from build123d import *

# Parameters (mm, degrees)
SKETCH1_W                    = 100
SKETCH1_H                    = 214.69
BASE_FLANGE1_DEPTH           = 0.81
EDGE_FLANGE1_STRIP_W         = 4.7132
EDGE_FLANGE1_STRIP_H         = 0.81
EDGE_FLANGE1_STRIP_CUT_DEPTH = 214.69
EDGE_FLANGE1_DEPTH           = 214.69
EDGE_FLANGE2_STRIP_W         = 4.7132
EDGE_FLANGE2_STRIP_H         = 0.81
EDGE_FLANGE2_STRIP_CUT_DEPTH = 214.69
EDGE_FLANGE2_DEPTH           = 214.69
EDGE_FLANGE3_DEPTH           = 98.4534
EDGE_FLANGE3_BEND_DEPTH      = 97.2634
SKETCH18_W                   = 29
SKETCH18_H                   = 1.5466
SKETCH18_W_2                 = 27
CUT_EXTRUDE1_DEPTH           = 23.81
CUT_EXTRUDE2_REACH           = 249.484
SKETCH19_R                   = 2.5
SKETCH19_R_2                 = 3.5
SKETCH19_R_3                 = 1.5
SKETCH19_R_4                 = 3.25
CUT_EXTRUDE3_REACH           = 249.484
SKETCH20_R                   = 1.85
SKETCH20_R_2                 = 2.5
SKETCH20_R_3                 = 3.5


# Sheet-metal steps are written as plain solids
with BuildPart() as part:
    # Sketch1 → Base-Flange1 (new body)
    with BuildSketch(Plane.XY):
        with Locations((50, 107.345)):
            Rectangle(SKETCH1_W, SKETCH1_H)
    extrude(amount=-BASE_FLANGE1_DEPTH)

    # Edge-Flange1 strip (across the edge) → Edge-Flange1 strip cut (cut)
    with BuildSketch(Plane(origin=(100, 214.69, -0.81), x_dir=(-1, 0, 0), z_dir=(0, -1, 0))):
        with Locations((-0.81, -0.405)):
            Rectangle(EDGE_FLANGE1_STRIP_W, EDGE_FLANGE1_STRIP_H)
    extrude(amount=EDGE_FLANGE1_STRIP_CUT_DEPTH, mode=Mode.SUBTRACT)

    # Edge-Flange1 section (across the edge) → Edge-Flange1 (add)
    with BuildSketch(Plane(origin=(100, 214.69, -0.81), x_dir=(-1, 0, 0), z_dir=(0, -1, 0))):
        with BuildLine():
            Line((0, 0.7366), (0, 48))
            Line((0, 48), (0.81, 48))
            Line((0.81, 48), (0.81, 0.7366))
            ThreePointArc((0.81, 0.7366), (1.025745145, 0.215745145), (1.5466, 0))
            Line((1.5466, 0), (1.5466, -0.81))
            ThreePointArc((1.5466, -0.81), (0.452988652, -0.357011348), (0, 0.7366))
        make_face()
    extrude(amount=EDGE_FLANGE1_DEPTH)

    # Edge-Flange2 strip (across the edge) → Edge-Flange2 strip cut (cut)
    with BuildSketch(Plane(origin=(99.19, 214.69, -48.81), x_dir=(0, 0, 1), z_dir=(0, -1, 0))):
        with Locations((-0.81, -0.405)):
            Rectangle(EDGE_FLANGE2_STRIP_W, EDGE_FLANGE2_STRIP_H)
    extrude(amount=EDGE_FLANGE2_STRIP_CUT_DEPTH, mode=Mode.SUBTRACT)

    # Edge-Flange2 section (across the edge) → Edge-Flange2 (add)
    with BuildSketch(Plane(origin=(99.19, 214.69, -48.81), x_dir=(0, 0, 1), z_dir=(0, -1, 0))):
        with BuildLine():
            Line((0, 0.7366), (0, 98))
            Line((0, 98), (0.81, 98))
            Line((0.81, 98), (0.81, 0.7366))
            ThreePointArc((0.81, 0.7366), (1.025745145, 0.215745145), (1.5466, 0))
            Line((1.5466, 0), (1.5466, -0.81))
            ThreePointArc((1.5466, -0.81), (0.452988652, -0.357011348), (0, 0.7366))
        make_face()
    extrude(amount=EDGE_FLANGE2_DEPTH)

    # Edge-Flange3 section (across the edge) → Edge-Flange3 (add)
    with BuildSketch(Plane(origin=(0, -0.7366, 0), x_dir=(0, 1, 0), z_dir=(1, 0, 0))):
        with BuildLine():
            Line((-0.81, 0.7366), (-0.81, 23))
            Line((-0.81, 23), (0, 23))
            Line((0, 23), (0, 0.7366))
            ThreePointArc((0, 0.7366), (0.215745145, 0.215745145), (0.7366, 0))
            Line((0.7366, 0), (0.7366, -0.81))
            ThreePointArc((0.7366, -0.81), (-0.357011348, -0.357011348), (-0.81, 0.7366))
        make_face()
    extrude(amount=EDGE_FLANGE3_DEPTH)

    # Edge-Flange3 section 2 (across the edge) → Edge-Flange3 bend (add)
    with BuildSketch(Plane(origin=(98.4534, -0.7366, -48.81), x_dir=(0, 1, 0), z_dir=(-1, 0, 0))):
        with BuildLine():
            Line((-0.81, 0.7366), (-0.81, 23))
            Line((-0.81, 23), (0, 23))
            Line((0, 23), (0, 0.7366))
            ThreePointArc((0, 0.7366), (0.215745145, 0.215745145), (0.7366, 0))
            Line((0.7366, 0), (0.7366, -0.81))
            ThreePointArc((0.7366, -0.81), (-0.357011348, -0.357011348), (-0.81, 0.7366))
        make_face()
    extrude(amount=EDGE_FLANGE3_BEND_DEPTH)

    # Sketch18 → Cut-Extrude1 (cut)
    with BuildSketch(Plane(origin=(0, -57.7366, -71.81), x_dir=(1, 0, 0), z_dir=(0, 0, 1))):
        with Locations((83.9534, 56.9633)):
            Rectangle(SKETCH18_W, SKETCH18_H)
        with Locations((14.69, 56.9633)):
            Rectangle(SKETCH18_W_2, SKETCH18_H)
    extrude(amount=CUT_EXTRUDE1_DEPTH, mode=Mode.SUBTRACT)

    # Sketch19 → Cut-Extrude2 (cut, up to next)
    with BuildSketch(Plane.XY.offset(-48.81), mode=Mode.PRIVATE) as cut_extrude2_sk1:
        with Locations((40, 199.69)):
            Circle(SKETCH19_R)
    cut_extrude2_tool1 = extrude(cut_extrude2_sk1.sketch, amount=CUT_EXTRUDE2_REACH, mode=Mode.PRIVATE) & part.part
    # Sketch19 → Cut-Extrude2 (cut, up to next)
    with BuildSketch(Plane.XY.offset(-48.81), mode=Mode.PRIVATE) as cut_extrude2_sk2:
        with Locations((10, 149.69)):
            Circle(SKETCH19_R)
    cut_extrude2_tool2 = extrude(cut_extrude2_sk2.sketch, amount=CUT_EXTRUDE2_REACH, mode=Mode.PRIVATE) & part.part
    # Sketch19 → Cut-Extrude2 (cut, up to next)
    with BuildSketch(Plane.XY.offset(-48.81), mode=Mode.PRIVATE) as cut_extrude2_sk3:
        with Locations((64.901247632, 149.252126171)):
            Circle(SKETCH19_R_2)
    cut_extrude2_tool3 = extrude(cut_extrude2_sk3.sketch, amount=CUT_EXTRUDE2_REACH, mode=Mode.PRIVATE) & part.part
    # Sketch19 → Cut-Extrude2 (cut, up to next)
    with BuildSketch(Plane.XY.offset(-48.81), mode=Mode.PRIVATE) as cut_extrude2_sk4:
        with Locations((64.901247632, 171.426326171)):
            Circle(SKETCH19_R_3)
    cut_extrude2_tool4 = extrude(cut_extrude2_sk4.sketch, amount=CUT_EXTRUDE2_REACH, mode=Mode.PRIVATE) & part.part
    # Sketch19 → Cut-Extrude2 (cut, up to next)
    with BuildSketch(Plane.XY.offset(-48.81), mode=Mode.PRIVATE) as cut_extrude2_sk5:
        with Locations((75.112047632, 149.252126171)):
            Circle(SKETCH19_R_3)
    cut_extrude2_tool5 = extrude(cut_extrude2_sk5.sketch, amount=CUT_EXTRUDE2_REACH, mode=Mode.PRIVATE) & part.part
    # Sketch19 → Cut-Extrude2 (cut, up to next)
    with BuildSketch(Plane.XY.offset(-48.81), mode=Mode.PRIVATE) as cut_extrude2_sk6:
        with Locations((54.690447632, 149.252126171)):
            Circle(SKETCH19_R_3)
    cut_extrude2_tool6 = extrude(cut_extrude2_sk6.sketch, amount=CUT_EXTRUDE2_REACH, mode=Mode.PRIVATE) & part.part
    # Sketch19 → Cut-Extrude2 (cut, up to next)
    with BuildSketch(Plane.XY.offset(-48.81), mode=Mode.PRIVATE) as cut_extrude2_sk7:
        with Locations((64.901247632, 122.577226171)):
            Circle(SKETCH19_R_4)
    cut_extrude2_tool7 = extrude(cut_extrude2_sk7.sketch, amount=CUT_EXTRUDE2_REACH, mode=Mode.PRIVATE) & part.part
    add(cut_extrude2_tool1.solids().sort_by_distance((40, 199.69, -48.81))[0], mode=Mode.SUBTRACT)
    add(cut_extrude2_tool2.solids().sort_by_distance((10, 149.69, -48.81))[0], mode=Mode.SUBTRACT)
    add(cut_extrude2_tool3.solids().sort_by_distance((64.901248, 149.252126, -48.81))[0], mode=Mode.SUBTRACT)
    add(cut_extrude2_tool4.solids().sort_by_distance((64.901248, 171.426326, -48.81))[0], mode=Mode.SUBTRACT)
    add(cut_extrude2_tool5.solids().sort_by_distance((75.112048, 149.252126, -48.81))[0], mode=Mode.SUBTRACT)
    add(cut_extrude2_tool6.solids().sort_by_distance((54.690448, 149.252126, -48.81))[0], mode=Mode.SUBTRACT)
    add(cut_extrude2_tool7.solids().sort_by_distance((64.901248, 122.577226, -48.81))[0], mode=Mode.SUBTRACT)

    # Sketch20 → Cut-Extrude3 (cut, up to next)
    with BuildSketch(Plane.XY, mode=Mode.PRIVATE) as cut_extrude3_sk1:
        with Locations((63.4534, 199.69)):
            Circle(SKETCH20_R)
    cut_extrude3_tool1 = extrude(cut_extrude3_sk1.sketch, amount=-CUT_EXTRUDE3_REACH, mode=Mode.PRIVATE) & part.part
    # Sketch20 → Cut-Extrude3 (cut, up to next)
    with BuildSketch(Plane.XY, mode=Mode.PRIVATE) as cut_extrude3_sk2:
        with Locations((10, 149.69)):
            Circle(SKETCH20_R_2)
    cut_extrude3_tool2 = extrude(cut_extrude3_sk2.sketch, amount=-CUT_EXTRUDE3_REACH, mode=Mode.PRIVATE) & part.part
    # Sketch20 → Cut-Extrude3 (cut, up to next)
    with BuildSketch(Plane.XY, mode=Mode.PRIVATE) as cut_extrude3_sk3:
        with Locations((64.901247632, 149.252126171)):
            Circle(SKETCH20_R_3)
    cut_extrude3_tool3 = extrude(cut_extrude3_sk3.sketch, amount=-CUT_EXTRUDE3_REACH, mode=Mode.PRIVATE) & part.part
    add(cut_extrude3_tool1.solids().sort_by_distance((63.4534, 199.69, 0))[0], mode=Mode.SUBTRACT)
    add(cut_extrude3_tool2.solids().sort_by_distance((10, 149.69, 0))[0], mode=Mode.SUBTRACT)
    add(cut_extrude3_tool3.solids().sort_by_distance((64.901248, 149.252126, 0))[0], mode=Mode.SUBTRACT)


solid = part.part
Design review of the part built by this model. Coordinates are the model's own, in mm. A direction names the side the tool comes from. Coordinates: 2 decimals unless noted, no trailing zeros. Order: outer loops, then holes, each group sorted by start corner. A loop starts at its lowest first (then second) coordinate and runs counter-clockwise, first axis right, second up. Notation, with made-up numbers: (-26.5, 45.25) -> (24.5, 45.25) arc R18 cw to (24.5, 56.25) -> close; hole circle Ø7 at (17, 35). An arc over 180 degrees is marked (long way). Use one line per item in the form item = value. Start each with the question number.
(1) For probe 1 along X at (y, z) = (149.69, -0.2); probe 2 along Z at (x, y) = (7, 18); probe 3 along X at (y, z) = (201.5, -27), list the stretches that pass through material, from the lowest coordinate up.
(2) Add section B-B on x = 86. State the section outline as (y, z) points.
(3) For faces 1 (the flat face through (99.19, 109, -25)), 2 (the flat face through (51, 109, -48.81)), 3 (the flat face through (99.4, 0, -35.4)), list the 3-axis set-ups (+Z, -Z, +X, -X, +Y, -Y) from which the entire face can be reached by the end or side of a thin tool; tool diameter is ignored.
(4) Add section A-A on x = 40. State the section outline as (y, z) points.
(5) The part is to be moulded in two halves that separate along Z. For faces 4 (the flat face through (0, 107.1, -0.3)), 5 (the flat face through (49, 109, -48)), 6 (the flat face through (49, 109, 0)), say which applies: +Z half, -Z half, draft (parallel to the pull), parting line (faces both ways), or undercut.
(6) Add section C-C on y = 106. State the section outline as (x, z) points, plus the area to 3 significant figures.
(7) Add section D-D on z = -61. State the section outline as (x, y) points.
(8) Insertion check: pin 1 (6 mm diameter, centred on x = 63.45, y = 199.69, fed in from -Z); pin 2 (2.5 mm diameter, centred on x = 75.11, y = 149.25, fed in from +Z); pin 3 (0.8 mm diameter, centred on y = -1, z = -57, fed in from +X). Each pin has a flat end and moves straight along its axis. Give the tip position at first contact, or say it passes through.
Answer block:
q1.probe_1 = 0 to 7.5, 12.5 to 61.43, 68.37 to 99.21
q1.probe_2 = -48.81 to -48, -0.81 to 0
q1.probe_3 = 99.19 to 100
q2.outline = (-1.55, 0.74) arc R1.55 ccw to (0, -0.81) -> (214.69, -0.81) -> (214.69, 0) -> (0, 0) arc R0.74 cw to (-0.74, 0.74) -> (-0.74, 23) -> (-1.55, 23) -> close; (0, -48.81) -> (214.69, -48.81) -> (214.69, -48) -> (0, -48) -> close
q3.face_1 = -X, +Y, -Y
q3.face_2 = -Z, +X, -X, +Y
q3.face_3 = -Z, +X, -Y
q4.outline = (-1.55, -71.81) -> (-0.74, -71.81) -> (-0.74, -49.55) arc R0.74 cw to (0, -48.81) -> (197.19, -48.81) -> (197.19, -48) -> (0, -48) arc R1.55 ccw to (-1.55, -49.55) -> close; (-1.55, 0.74) arc R1.55 ccw to (0, -0.81) -> (214.69, -0.81) -> (214.69, 0) -> (0, 0) arc R0.74 cw to (-0.74, 0.74) -> (-0.74, 23) -> (-1.55, 23) -> close; (202.19, -48.81) -> (214.69, -48.81) -> (214.69, -48) -> (202.19, -48) -> close
q5.face_4 = draft
q5.face_5 = undercut
q5.face_6 = +Z half
q6.outline = (0, -0.81) -> (98.45, -0.81) arc R0.74 cw to (99.19, -1.55) -> (99.19, -47.26) arc R0.74 cw to (98.45, -48) -> (1.19, -48) -> (1.19, -48.81) -> (98.45, -48.81) arc R1.55 ccw to (100, -47.26) -> (100, -1.55) arc R1.55 ccw to (98.45, 0) -> (0, 0) -> close
q6.area = 198 mm²
q7.outline = (28.19, -1.55) -> (69.45, -1.55) -> (69.45, -0.74) -> (28.19, -0.74) -> close
q8.pin_1 = -48.81
q8.pin_2 = 0
q8.pin_3 = 69.45
